Work out the finished part from the listing and answer in its coordinate system (mm). Give positions to 0.01 mm unless a question says otherwise; leave off trailing zeros. Loops run counter-clockwise (first coordinate to the right, second up) from the corner with the lowest first, then second, coordinate; pieces in that order, holes last.
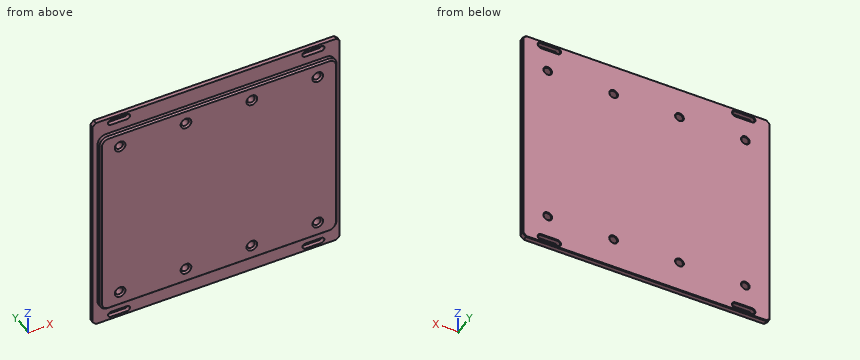
```python
from build123d import *

# Parameters (mm, degrees)
SKETCH027_W     = 75
SKETCH027_H     = 138.2
PAD016_DEPTH    = 3
POCKET012_DEPTH = 5
CHAMFER016_SIZE = 2
SKETCH029_W     = 144
SKETCH029_H     = 118.2
PAD017_DEPTH    = 3
FILLET005_R     = 5
SKETCH030_R     = 2.25
POCKET013_DEPTH = 7
CHAMFER017_SIZE = 1
CHAMFER018_SIZE = 0.4


with BuildPart() as part:
    # Sketch027 (on XZ_Plane007 of Origin028) → Pad016 (new body)
    with BuildSketch(Plane.XZ):
        with Locations((37.5, 0)):
            Rectangle(SKETCH027_W, SKETCH027_H)
    extrude(amount=PAD016_DEPTH)

    # Sketch028 (on XZ_Plane007 of Origin028) → Pocket012 (cut)
    with BuildSketch(Plane.XZ):
        with BuildLine():
            ThreePointArc((64, 64.3), (65.7, 66), (64, 67.7))
            Line((64, 67.7), (54, 67.7))
            ThreePointArc((54, 67.7), (52.3, 66), (54, 64.3))
            Line((64, 64.3), (54, 64.3))
        make_face()
    pocket012 = extrude(amount=POCKET012_DEPTH, mode=Mode.SUBTRACT)

    # Mirrored010: Pocket012 across XY
    add(pocket012.mirror(Plane.XY), mode=Mode.SUBTRACT)

    # Mirrored011: part across YZ


with BuildPart() as part_1:
    add(part.part)
    add(part.part.mirror(Plane.YZ))

    # Chamfer016
    chamfer016_edges = [part_1.edges().sort_by_distance(p)[0] for p in [
        (-75, -1.5, -69.1),
        (75, -1.5, -69.1),
        (-75, -1.5, 69.1),
        (75, -1.5, 69.1),
    ]]
    chamfer(chamfer016_edges, length=CHAMFER016_SIZE)

    # Sketch029 (on Face5 of Chamfer016) → Pad017 (join)
    with BuildSketch(Plane.XZ.offset(3)):
        Rectangle(SKETCH029_W, SKETCH029_H)
    extrude(amount=PAD017_DEPTH)

    # Fillet005
    fillet005_edges = [part_1.edges().sort_by_distance(p)[0] for p in [
        (72, -4.5, -59.1),
        (72, -4.5, 59.1),
        (-72, -4.5, -59.1),
        (-72, -4.5, 59.1),
    ]]
    fillet(fillet005_edges, radius=FILLET005_R)

    # Sketch030 (on Face34 of Fillet005) → Pocket013 (cut)
    with BuildSketch(Plane.XZ.offset(6)):
        with Locations((-60, 50)):
            Circle(SKETCH030_R)
        with Locations((-20, 50)):
            Circle(SKETCH030_R)
        with Locations((20, 50)):
            Circle(SKETCH030_R)
        with Locations((60, 50)):
            Circle(SKETCH030_R)
        with Locations((60, -50)):
            Circle(SKETCH030_R)
        with Locations((20, -50)):
            Circle(SKETCH030_R)
        with Locations((-20, -50)):
            Circle(SKETCH030_R)
        with Locations((-60, -50)):
            Circle(SKETCH030_R)
    extrude(amount=-POCKET013_DEPTH, mode=Mode.SUBTRACT)

    # Chamfer017
    chamfer017_edges = [part_1.edges().sort_by_distance(p)[0] for p in [
        (0, -6, -59.1),
        (-70.535534, -6, -57.635534),
        (70.535534, -6, -57.635534),
        (-72, -6, 0),
        (72, -6, 0),
        (-70.535534, -6, 57.635534),
        (70.535534, -6, 57.635534),
        (0, -6, 59.1),
        (-62.25, -6, -50),
        (-22.25, -6, -50),
        (-62.25, -6, 50),
        (-22.25, -6, 50),
        (17.75, -6, -50),
        (57.75, -6, -50),
        (17.75, -6, 50),
        (57.75, -6, 50),
    ]]
    chamfer(chamfer017_edges, length=CHAMFER017_SIZE)

    # Chamfer018
    chamfer018_edges = [part_1.edges().sort_by_distance(p)[0] for p in [
        (0, 0, -69.1),
        (74, 0, -68.1),
        (-74, 0, -68.1),
        (75, 0, 0),
        (-75, 0, 0),
        (74, 0, 68.1),
        (-74, 0, 68.1),
        (0, 0, 69.1),
        (-65.7, 0, -66),
        (-59, 0, -64.3),
        (-59, 0, -67.7),
        (-52.3, 0, -66),
        (-62.25, 0, -50),
        (-22.25, 0, -50),
        (-62.25, 0, 50),
        (-59, 0, 64.3),
        (-65.7, 0, 66),
        (-52.3, 0, 66),
        (-59, 0, 67.7),
        (-22.25, 0, 50),
        (17.75, 0, -50),
        (65.7, 0, -66),
        (59, 0, -64.3),
        (59, 0, -67.7),
        (52.3, 0, -66),
        (57.75, 0, -50),
        (17.75, 0, 50),
        (57.75, 0, 50),
        (59, 0, 64.3),
        (65.7, 0, 66),
        (52.3, 0, 66),
        (59, 0, 67.7),
    ]]
    chamfer(chamfer018_edges, length=CHAMFER018_SIZE)


solid = part_1.part
```
Q1. Section C-C on z = 50 is taken. State how many separate pieces and enclosed holes the cut face has, plus the area to 3 significant figures.
Q2. Consider line 1 along Z through (x, y) = (20, -2.2); line 2 along Z through (x, y) = (60, -2.75); line 3 along X through (y, z) = (-0.75, -51). Determine where each line is inside the solid, lowest interval first.
Q3. Section A-A on x = -47 is taken. Give the vertices of the cut face in (y, z), plus the area to 3 significant figures.
Q4. Section B-B on z = -12 is taken. Give the vertices of the cut face in (x, y), plus the area to 3 significant figures.
Q5. Given pin 1 (4 mm diameter, centred on x = -60, z = -50, fed in from +Y); pin 2 (1 mm diameter, centred on x = -22.5, y = -4, fed in from -Z); pin 3 (0.6 mm diameter, centred on y = -4.5, z = -0.5, fed in from -X), each flat-ended and moving along its own axis, determine where each tip first touches the part or whether it passes through.
Check result:
1. separate pieces: 5
1. enclosed holes: 0
1. area: 768 mm2
2. line 1: z = -69.1 to -52.25, -47.75 to 47.75, 52.25 to 69.1
2. line 2: z = -69.1 to -67.7, -64.3 to -52.25, -47.75 to 47.75, 52.25 to 64.3, 67.7 to 69.1
2. line 3: x = -75 to -62.02, -57.98 to -22.02, -17.98 to 17.98, 22.02 to 57.98, 62.02 to 75
3. outline: (-6, -58.1) - (-5, -59.1) - (-3, -59.1) - (-3, -69.1) - (-0.4, -69.1) - (0, -68.7) - (0, 68.7) - (-0.4, 69.1) - (-3, 69.1) - (-3, 59.1) - (-5, 59.1) - (-6, 58.1) - close
3. area: 768 mm2
4. outline: (-75, -3) - (-72, -3) - (-72, -5) - (-71, -6) - (71, -6) - (72, -5) - (72, -3) - (75, -3) - (75, -0.4) - (74.6, 0) - (-74.6, 0) - (-75, -0.4) - close
4. area: 881 mm2
5. pin 1: passes through
5. pin 2: stops at z = -59.1
5. pin 3: stops at x = -72
